Check sheet for the modelled part. Datum: model origin and axes. Units: mm. A direction names the side the tool comes from. Round coordinates to 2 decimals unless told otherwise and drop trailing zeros. Write each loop counter-clockwise with the first axis right and the second up, starting at its lowest first coordinate (ties: lowest second). Pieces come first, ordered by that corner, then holes. Notation, with made-up numbers: (52, 25) - (91, 25) arc R8 ccw to (91, 30) - close; hole circle Ø5 at (-24, 52.5). An arc over 180 degrees is marked (long way). Answer as a JSON object with one key per item and string values. Group by question number.
Item 1: Set-up check for faces 5 (the flat face through (-11.22, 2.74, 22.53)), 6 (the flat face through (0, 0, 21)), 7 (the flat face through (-9.25, 1, 25)), 8 (the cylindrical face through (14.87, 6.13, 9.71)), 9 (the flat face through (9.25, 1, -6)): record each of +Z, -Z, +X, -X, +Y, -Y from which the full face is reachable in a straight line by a thin tool's end or side.
Item 2: Thickness scan on line 1 (X direction, y = 1, z = 9.5); line 2 (Z direction, x = 5.5, y = 0.5); line 3 (X direction, y = 7, z = 8.5). Record the ranges inside material, lowest first.
Item 3: Sectioned sample at A-A on x = 8. Record the boundary of the cut face in (y, z).
Item 4: Sectioned sample at C-C on x = 0. Record the boundary of the cut face in (y, z).
Item 5: Sectioned sample at B-B on z = 19.5. Record the boundary of the cut face in (x, y), plus the area to 3 significant figures.
Item 6: Gauge pin test, flat ends, axial feed: P1, Ø1.5, axis at y = 2.5, z = 2.5, coming from the -X side; P2, Ø4.5, axis at x = 3, z = 22.5, coming from the +Y side; P3, Ø1.2, axis at y = 1, z = 25.5, coming from the -X side. Record the tip position at first contact, or that the pin passes through.
Item 7: Sectioned sample at D-D on x = -11.5. Record the boundary of the cut face in (y, z).
Item 8: Release check for a two-part mould opening along Z. For faces 1 (the flat face through (-20, 1, -1.5)), 2 (the flat face through (20.28, 2.74, 22.53)), 3 (the flat face through (6.18, 0.99, -5.48)), 4 (the flat face through (-7, 1, 26)) record: pulls with the +Z half, pulls with the -Z half, needs draft (parallel to the pull), parting line crosses it, or undercut.
```python
from build123d import *

# Parameters (mm, degrees)
SKETCH_1_W               = 4
SKETCH_1_H               = 11
SKETCH_1_H_2             = 8
EXTRUDE_1_DEPTH          = 4
SKETCH_1_7_W             = 44.5
SKETCH_1_7_H             = 8
EXTRUDE_2_DEPTH          = 3.5
SKETCH_2_W               = 18.5
SKETCH_2_H               = 1.5
CUT_EXTRUDE_1_DEPTH      = 30.53070436
SKETCH_2_3_W             = 2.5
SKETCH_2_3_H             = 1.5
EXTRUDE_4_DEPTH          = 19
FILLET_1_R               = 1
FILLET_2_R               = 1.5
FILLET_3_R               = 1
CUT_EXTRUDE_2_DEPTH      = 37.65122781
CUT_EXTRUDE_2_DEPTH_BACK = 37.65122781


with BuildPart() as part:
    # 草图1 → 凸台-拉伸1 (new body)
    with BuildSketch(Plane(origin=(0, 0, 0), x_dir=(1, 0, 0), z_dir=(0, 1, 0))):
        with Locations((-15.75, -4)):
            Rectangle(SKETCH_1_W, SKETCH_1_H)
        with Locations((15.75, -4)):
            Rectangle(SKETCH_1_W, SKETCH_1_H)
        with Locations((15.75, 5.5)):
            Rectangle(SKETCH_1_W, SKETCH_1_H_2)
        with Locations((-15.75, 5.5)):
            Rectangle(SKETCH_1_W, SKETCH_1_H_2)
    extrude(amount=EXTRUDE_1_DEPTH)

    # 草图1<7> → 凸台-拉伸2 (add)
    with BuildSketch(Plane(origin=(0, 0, 0), x_dir=(1, 0, 0), z_dir=(0, 1, 0))):
        with Locations((0, 5.5)):
            Rectangle(SKETCH_1_7_W, SKETCH_1_7_H)
    extrude(amount=EXTRUDE_2_DEPTH)

    # 草图2 → 切除-拉伸1 (cut, through all)
    with BuildSketch(Plane(origin=(0, 0, -9.5), x_dir=(-1, 0, 0), z_dir=(0, 0, -1))):
        with Locations((0, 2.75)):
            Rectangle(SKETCH_2_W, SKETCH_2_H)
        Polygon((13.25, 3.5), (9.25, 3.5), (9.25, 2), align=None)
        Polygon((-9.25, 3.5), (-13.25, 3.5), (-9.25, 2), align=None)
        Polygon((-22.25, 3.5), (-22.25, 2), (-18.25, 3.5), align=None)
        Polygon((22.25, 3.5), (18.25, 3.5), (22.25, 2), align=None)
    extrude(amount=-CUT_EXTRUDE_1_DEPTH, mode=Mode.SUBTRACT)

    # 草图2<3> → 凸台-拉伸4 (add, through all)
    with BuildSketch(Plane(origin=(0, 0, -9.5), x_dir=(-1, 0, 0), z_dir=(0, 0, -1))):
        with Locations((-15.75, 7.25)):
            Rectangle(SKETCH_2_3_W, SKETCH_2_3_H)
        Polygon((-15, 6.5), (-16.5, 6.5), (-16.5, 4), (-15.75, 4), (-15, 4), align=None)
        with Locations((15.75, 7.25)):
            Rectangle(SKETCH_2_3_W, SKETCH_2_3_H)
        Polygon((16.5, 6.5), (15, 6.5), (15, 4), (15.75, 4), (16.5, 4), align=None)
    extrude(amount=-EXTRUDE_4_DEPTH)

    # 圆角1
    # the kernel refuses this fillet: 1 mm, written as the material it adds along each edge
    with BuildSketch(Plane(origin=(-16.5, 6.5, -9.5), x_dir=(0, -1, 0), z_dir=(0, 0, 1))) as fillet_1_piece_1:
        with BuildLine():
            CenterArc((0.866025404, -1), FILLET_1_R, 90, 60)
            Line((0, -0.5), (-0.017320508, -0.49))
            ThreePointArc((-0.017320508, -0.49), (-0.02, -0.25), (-0.02, 0))
            Line((-0.02, 0), (0, 0.02))
            Line((0, 0.02), (0.866025404, 0.02))
            Line((0.866025404, 0.02), (0.866025404, 0))
        make_face()
    extrude(amount=19)
    with BuildSketch(Plane(origin=(-15, 6.5, -9.5), x_dir=(0, -1, 0), z_dir=(0, 0, 1)), Plane(origin=(16.5, 6.5, -9.5), x_dir=(0, -1, 0), z_dir=(0, 0, 1))) as fillet_1_piece_2:
        with BuildLine():
            CenterArc((0.866025404, 1), FILLET_1_R, 210, 60)
            Line((0, 0.5), (-0.017320508, 0.49))
            ThreePointArc((-0.017320508, 0.49), (-0.02, 0.25), (-0.02, 0))
            Line((-0.02, 0), (0, -0.02))
            Line((0, -0.02), (0.866025404, -0.02))
            Line((0.866025404, -0.02), (0.866025404, 0))
        make_face()
    extrude(amount=19)
    with BuildSketch(Plane(origin=(15, 6.5, -9.5), x_dir=(-1, 0, 0), z_dir=(0, 0, 1))) as fillet_1_piece_3:
        with BuildLine():
            CenterArc((1, 0.866025404), FILLET_1_R, 180, 60)
            Line((0, 0.866025404), (-0.02, 0.866025404))
            Line((-0.02, 0.866025404), (-0.02, 0))
            Line((-0.02, 0), (0, -0.02))
            ThreePointArc((0, -0.02), (0.25, -0.02), (0.49, -0.017320508))
            Line((0.49, -0.017320508), (0.5, 0))
        make_face()
    extrude(amount=19)

    # 圆角2
    # the kernel refuses this fillet: 1.5 mm, written as the material it adds along each edge
    with BuildSketch(Plane(origin=(16.5, 4, -9.5), x_dir=(1, 0, 0), z_dir=(0, 0, 1)), Plane(origin=(-15, 4, -9.5), x_dir=(1, 0, 0), z_dir=(0, 0, 1))) as fillet_2_piece_1:
        with BuildLine():
            CenterArc((1.5, 1.479019946), FILLET_2_R, 180, 80.405931773)
            Line((0, 1.479019946), (-0.03, 1.479019946))
            Line((-0.03, 1.479019946), (-0.03, 0))
            Line((-0.03, 0), (0, -0.03))
            ThreePointArc((0, -0.03), (0.625, -0.03), (1.245, -0.029580399))
            Line((1.245, -0.029580399), (1.25, 0))
        make_face()
    extrude(amount=19)
    with BuildSketch(Plane(origin=(15, 4, -9.5), x_dir=(0, 1, 0), z_dir=(0, 0, 1)), Plane(origin=(-16.5, 4, -9.5), x_dir=(0, 1, 0), z_dir=(0, 0, 1))) as fillet_2_piece_2:
        with BuildLine():
            CenterArc((1.479019946, 1.5), FILLET_2_R, 189.594068227, 80.405931773)
            Line((0, 1.25), (-0.029580399, 1.245))
            ThreePointArc((-0.029580399, 1.245), (-0.03, 0.625), (-0.03, 0))
            Line((-0.03, 0), (0, -0.03))
            Line((0, -0.03), (1.479019946, -0.03))
            Line((1.479019946, -0.03), (1.479019946, 0))
        make_face()
    extrude(amount=19)

    # 圆角3
    fillet_3_edges = [part.edges().sort_by_distance(p)[0] for p in [
        (14.5, 8, 0),
        (17, 8, 0),
        (-17, 8, 0),
        (-14.5, 8, 0),
    ]]
    fillet(fillet_3_edges, radius=FILLET_3_R)

    # 镜向2: part across plane


with BuildPart() as part_1:
    add(part.part)
    add(part.part.mirror(Plane(origin=(0, 4, 9.5), x_dir=(1, 0, 0), z_dir=(0, 0, -1))))

    # 草图9 → 切除-拉伸2 (cut, two sides: drawn at the far end of the back side and taken through both)
    with BuildSketch(Plane(origin=(0, 2, 0), x_dir=(1, 0, 0), z_dir=(0, 1, 0)).offset(-CUT_EXTRUDE_2_DEPTH_BACK)):
        Polygon((-22.25, 5.5), (-9.25, 5.5), (-9.25, 4), (-5.25, 4), (-7.083333333, 7), (0.916666667, 7), (-0.916666667, 4), (7.083333333, 4), (5.25, 7), (9.25, 7), (9.25, 5.5), (22.25, 5.5), (22.25, 9.5), (-22.25, 9.5), align=None)
        Polygon((-22.25, -24.5), (-9.25, -24.5), (-9.25, -26), (-5.25, -26), (-7.083333333, -23), (0.916666667, -23), (-0.916666667, -26), (7.083333333, -26), (5.25, -23), (9.25, -23), (9.25, -24.5), (22.25, -24.5), (22.25, -28.5), (-22.25, -28.5), align=None)
    extrude(amount=CUT_EXTRUDE_2_DEPTH + CUT_EXTRUDE_2_DEPTH_BACK, mode=Mode.SUBTRACT)


solid = part_1.part
```
Completed:
{
 "1": {"face 5": "+Z, -Z, +Y", "face 6": "+Z, -Z, +X, -X, -Y", "face 7": "+Z, -X, +Y, -Y", "face 8": "+Z, -Z", "face 9": "-Z, +X, +Y, -Y"},
 "2": {"line 1": "-17.75 to -13.75, 13.75 to 17.75", "line 2": "-7 to -6.59, -4 to -1.5, 20.5 to 23, 23.41 to 26", "line 3": "-17 to -14.5, 14.5 to 17"},
 "3": {"outline": "(0, -7) - (2, -7) - (2, -1.5) - (0, -1.5) - close; (0, 20.5) - (2, 20.5) - (2, 23) - (0, 23) - close"},
 "4": {"outline": "(0, -7) - (2, -7) - (2, -5.5) - (0, -5.5) - close; (0, -4) - (2, -4) - (2, -1.5) - (0, -1.5) - close; (0, 20.5) - (2, 20.5) - (2, 23) - (0, 23) - close; (0, 24.5) - (2, 24.5) - (2, 26) - (0, 26) - close"},
 "5": {"outline": "(-17.75, 0) - (-13.75, 0) - (-13.75, 4) arc R1.5 cw to (-15, 5.48) - (-15, 5.63) arc R1 cw to (-14.5, 6.5) - (-14.5, 7) arc R1 ccw to (-15.5, 8) - (-16, 8) arc R1 ccw to (-17, 7) - (-17, 6.5) arc R1 cw to (-16.5, 5.63) - (-16.5, 5.48) arc R1.5 cw to (-17.75, 4) - close; (13.75, 0) - (17.75, 0) - (17.75, 4) arc R1.5 cw to (16.5, 5.48) - (16.5, 5.63) arc R1 cw to (17, 6.5) - (17, 7) arc R1 ccw to (16, 8) - (15.5, 8) arc R1 ccw to (14.5, 7) - (14.5, 6.5) arc R1 cw to (15, 5.63) - (15, 5.48) arc R1.5 cw to (13.75, 4) - close", "area": "48.5 mm²"},
 "6": {"P1": "x = -17.75", "P2": "y = 2", "P3": "x = -9.25"},
 "7": {"outline": "(0, -5.5) - (2.84, -5.5) - (2.84, -1.5) - (0, -1.5) - close; (0, 20.5) - (2.84, 20.5) - (2.84, 24.5) - (0, 24.5) - close"},
 "8": {"face 1": "undercut", "face 2": "needs draft", "face 3": "undercut", "face 4": "pulls with the +Z half"}
}
